Source: CAD feature listing. Evaluate the final solid. Frame: model axes, mm. A direction names the side the tool comes from. Coordinates: 2 decimals unless noted, no trailing zeros. Write each loop counter-clockwise with the first axis right and the second up, starting at its lowest first coordinate (ties: lowest second). Pieces come first, ordered by that corner, then holes. Notation, with made-up numbers: (54, 58) - (83, 58) arc R16 cw to (83, 89) - close; hole circle Ø7 at (43.5, 66.5). An arc over 180 degrees is marked (long way). One line per question, with ' | ' between items. Start each with the question number.
Q1. Line query: line 1 (Z direction, x = 0, y = 8.75); line 2 (Y direction, x = -5, z = 28); line 3 (Y direction, x = -9.25, z = 10). Output: solid intervals per line, ascending.
Q2. Contact query for a flat-ended pin moving along its axis: P1, Ø3, axis at x = 0, z = 50, coming from the -Y side. Output: stop coordinate, or through.
Q3. Cut plane A-A, the plane y = 5.75. Return loops of the section in (x, z), plus the area to 3 significant figures.
Q4. Cut plane B-B, the plane z = 50. Return loops of the section in (x, y).
Q5. Draft query along Z for faces 1 (the face through (-9, 0, 0)), 2 (the face through (-9, 0, 80)), 3 (the face through (-8.986, 0.601, 28.092)), 4 (the face through (10, 0, 39)). Return one class per face: +Z half, -Z half, draft (parallel to the pull), parting line (faces both ways), or undercut.
Q6. Access query for faces 5 (the face through (9, -1.2, 11.6)), 6 (the face through (-8, 0, 39)). Directions: +Z, -Z, +X, -X, +Y, -Y. A direction counts if a zero-diameter tool reaches every point of the face in a straight line with its end or side. Return the directions, or none.
Q7. Cut plane D-D, the plane y = 0. Return loops of the section in (x, z), plus the area to 3 significant figures.
```python
from build123d import *

# Parameters (mm, degrees)
SKETCH_1_W          = 20
SKETCH_1_H          = 20
SKETCH_1_W_2        = 16
SKETCH_1_H_2        = 16
EXTRUDE_1_DEPTH     = 80
SKETCH_2_R          = 2
CUT_EXTRUDE_1_DEPTH = 100
SKETCH_3_R          = 2
CUT_EXTRUDE_2_DEPTH = 100


with BuildPart() as part:
    # 草图1 → 凸台-拉伸1 (new body)
    with BuildSketch(Plane.XY):
        Rectangle(SKETCH_1_W, SKETCH_1_H)
        Rectangle(SKETCH_1_W_2, SKETCH_1_H_2, mode=Mode.SUBTRACT)
    extrude(amount=EXTRUDE_1_DEPTH)

    # 草图2 → 切除-拉伸1 (cut)
    with BuildSketch(Plane(origin=(10, 0, 0), x_dir=(0, 0, -1), z_dir=(1, 0, 0))):
        with Locations((-10, 0)):
            Circle(SKETCH_2_R)
        with Locations((-30, 0)):
            Circle(SKETCH_2_R)
    extrude(amount=-CUT_EXTRUDE_1_DEPTH, mode=Mode.SUBTRACT)

    # 草图3 → 切除-拉伸2 (cut)
    with BuildSketch(Plane.XZ.offset(10)):
        with Locations((0, 50)):
            Circle(SKETCH_3_R)
        with Locations((0, 70)):
            Circle(SKETCH_3_R)
    extrude(amount=-CUT_EXTRUDE_2_DEPTH, mode=Mode.SUBTRACT)


solid = part.part
```
Reply:
1) line 1: z = 0 to 48, 52 to 68, 72 to 80 | line 2: y = -10 to -8, 8 to 10 | line 3: y = -10 to -2, 2 to 10
2) P1: passes through
3) outline: (-10, 0) - (-8, 0) - (-8, 80) - (-10, 80) - close; (8, 0) - (10, 0) - (10, 80) - (8, 80) - close | area: 320 mm^2
4) outline: (-10, -10) - (-2, -10) - (-2, -8) - (-8, -8) - (-8, 8) - (-2, 8) - (-2, 10) - (-10, 10) - close; (2, -10) - (10, -10) - (10, 10) - (2, 10) - (2, 8) - (8, 8) - (8, -8) - (2, -8) - close
5) face 1: -Z half | face 2: +Z half | face 3: undercut | face 4: draft
6) face 5: +X, -X | face 6: +Z, -Z
7) outline: (-10, 0) - (-8, 0) - (-8, 8) - (-10, 8) - close; (-10, 12) - (-8, 12) - (-8, 28) - (-10, 28) - close; (-10, 32) - (-8, 32) - (-8, 80) - (-10, 80) - close; (8, 0) - (10, 0) - (10, 8) - (8, 8) - close; (8, 12) - (10, 12) - (10, 28) - (8, 28) - close; (8, 32) - (10, 32) - (10, 80) - (8, 80) - close | area: 288 mm^2
